Design review of the part shown in the three views and the two pictorial views. Dimensions are in mm from the part's minimum x, y and z. A direction names the side the tool comes from. Round coordinates to 2 decimals unless told otherwise and drop trailing zeros. Order: outer loops, then holes, each group sorted by start corner. A loop starts at its lowest first (then second) coordinate and runs counter-clockwise, first axis right, second up. Notation, with made-up numbers: M 74.5,72 L 124.5,72 A17 ccw 124.5,77 Z; hole C -15.75,38 d6. An arc over 180 degrees is marked long. Write item = value, one per line. Start each with the question number.
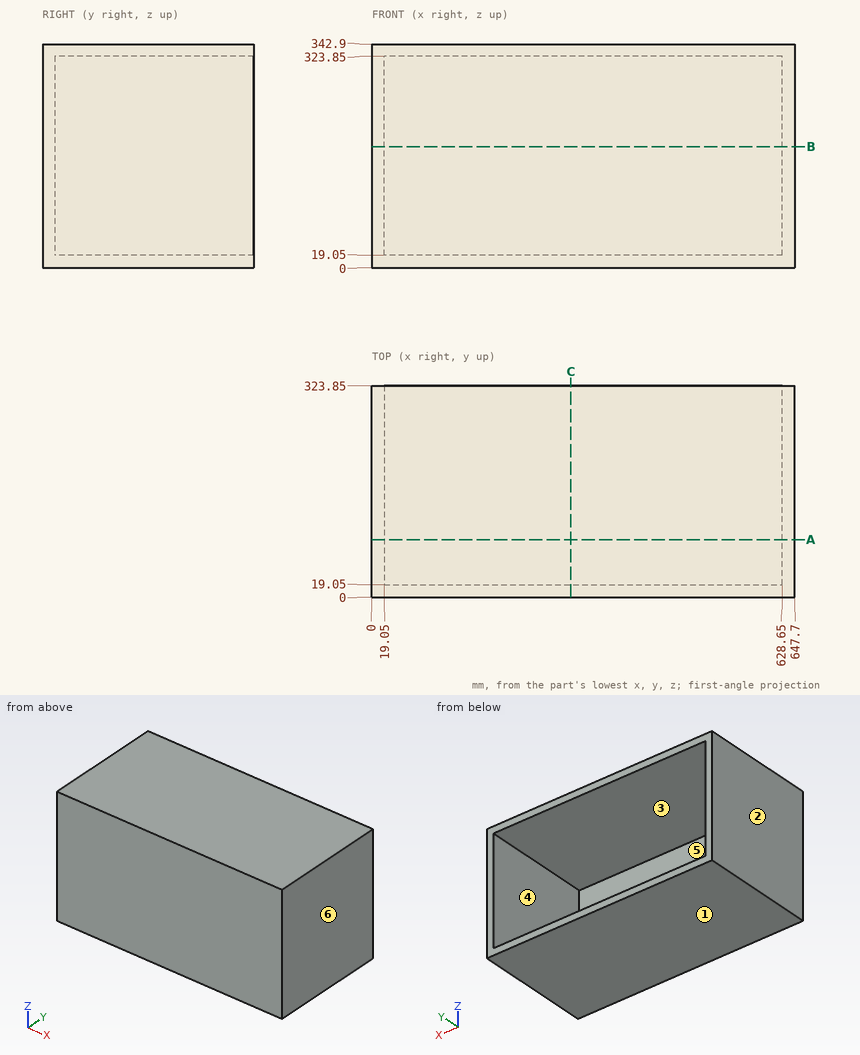
(1) Draft analysis for pull direction Z (two halves, no side actions). For the marked faces 1, 2, 3 and 4, state which applies: released by +Z, released by -Z, zero draft, split by the parting line, or undercut.
(2) We need section B-B, the plane z = 185.5. Write out the cut boundary in (x, y).
(3) We need section C-C, the plane x = 305. Write out the cut boundary in (y, z).
(4) For line 1 along X through (y, z) = (247, 203.5); line 2 along Z through (x, y) = (105, 209.5); line 3 along Y through (x, z) = (550, 40.5), list the stretches that pass through material, from the lowest coordinate up.
(5) Insertion check: pin 1 (5 mm diameter, centred on x = 442.5, y = 207.5, fed in from -Z); pin 2 (8 mm diameter, centred on x = 177, z = 243.5, fed in from +Y). Each pin has a flat end and moves straight along its axis. Give the tip position at first contact, or say it passes through.
(6) For the marked faces 5 and 6, list the 3-axis set-ups (+Z, -Z, +X, -X, +Y, -Y) from which the entire face can be reached by the end or side of a thin tool; tool diameter is ignored.
(7) We need section A-A, the plane y = 88. Write out the cut boundary in (x, z), then the cut area to 3 significant figures.
Values:
q1.face_1 = released by -Z
q1.face_2 = zero draft
q1.face_3 = undercut
q1.face_4 = undercut
q2.outline = M 0,0 L 647.7,0 L 647.7,323.85 L 628.65,323.85 L 628.65,19.05 L 19.05,19.05 L 19.05,323.85 L 0,323.85 Z
q3.outline = M 0,0 L 323.85,0 L 323.85,19.05 L 19.05,19.05 L 19.05,323.85 L 323.85,323.85 L 323.85,342.9 L 0,342.9 Z
q4.line_1 = 0 to 19.05, 628.65 to 647.7
q4.line_2 = 0 to 19.05, 323.85 to 342.9
q4.line_3 = 0 to 19.05
q5.pin_1 = 0
q5.pin_2 = 19.05
q6.face_5 = +Y
q6.face_6 = +Z, -Z, +X, +Y, -Y
q7.outline = M 0,0 L 647.7,0 L 647.7,342.9 L 0,342.9 Z; hole M 19.05,19.05 L 628.65,19.05 L 628.65,323.85 L 19.05,323.85 Z
q7.area = 36,300 mm²
